from build123d import *

# Parameters (mm, degrees)
ESQUISSE1_W        = 30
ESQUISSE1_H        = 140
ESQUISSE1_H_2      = 30
ESQUISSE1_W_2      = 350
BOSS_EXTRU_1_DEPTH = 580


with BuildPart() as part:
    # Esquisse1 → Boss.-Extru.1 (new body)
    with BuildSketch(Plane.XY):
        with Locations((-15, 100)):
            Rectangle(ESQUISSE1_W, ESQUISSE1_H)
        with Locations((-15, 15)):
            Rectangle(ESQUISSE1_W, ESQUISSE1_H_2)
        with Locations((175, 15)):
            Rectangle(ESQUISSE1_W_2, ESQUISSE1_H_2)
        with Locations((365, 15)):
            Rectangle(ESQUISSE1_W, ESQUISSE1_H_2)
        with Locations((365, 100)):
            Rectangle(ESQUISSE1_W, ESQUISSE1_H)
        Polygon((-30, 170), (-30, 152.681524316), (-15, 161.340762158), align=None)
        Polygon((-15, 161.340762158), (0, 170), (-30, 170), align=None)
        Polygon((-15, 161.340762158), (0, 152.681524316), (0, 170), align=None)
        Polygon((380, 170), (350, 170), (380, 152.681524316), align=None)
    extrude(amount=BOSS_EXTRU_1_DEPTH)


solid = part.part
Source: CAD feature listing. Evaluate the final solid. Frame: model axes, mm. A direction names the side the tool comes from. Coordinates: 2 decimals unless noted, no trailing zeros. Loops run counter-clockwise (first coordinate to the right, second up) from the corner with the lowest first, then second, coordinate; pieces in that order, holes last. Notation, with made-up numbers: (73.25, 7.25) - (99.25, 7.25) arc R7 ccw to (99.25, 13.25) - close; hole circle Ø1 at (62.25, 89.25). An arc over 180 degrees is marked (long way). One line per item, written item: value. Start each with the question number.
1. Contact query for flat-ended pins moving along their axis: P1, Ø3, axis at x = 118, z = 443.5, coming from the -Y side; P2, Ø6, axis at x = 302, z = 151, coming from the +Y side; P3, Ø10, axis at x = 25.5, y = 36, coming from the +Z side. Output: stop coordinate, or through.
2. Set-up query: faces 1 (the flat face through (365, 170, 286)), 2 (the flat face through (177, 30, 286)). Return all of +Z, -Z, +X, -X, +Y, -Y with unobstructed straight access to the full face (end or side cutting, diameter ignored); none if empty.
3. Section C-C (x = 108.5). Return the cut outline in (y, z), and give its area (3 significant figures).
4. Ray query, L1, parallel to X at y = 68, z = 544.5; L2, parallel to Y at x = 196.5, z = 182. Return the intervals inside material, ascending.
5. Section A-A (y = 139). Return the cut outline in (x, z), and give its area (3 significant figures).
6. Section B-B (z = 335). Return the cut outline in (x, y), and give its area (3 significant figures).
Verdict:
1. P1: stops at y = 0
1. P2: stops at y = 30
1. P3: passes through
2. face 1: +Z, -Z, +X, -X, +Y
2. face 2: +Z, -Z, +Y
3. outline: (0, 0) - (30, 0) - (30, 580) - (0, 580) - close
3. area: 17,400 mm2
4. L1: x = -30 to 0, 350 to 380
4. L2: y = 0 to 30
5. outline: (-30, 0) - (0, 0) - (0, 580) - (-30, 580) - close; (350, 0) - (380, 0) - (380, 580) - (350, 580) - close
5. area: 34,800 mm2
6. outline: (-30, 0) - (380, 0) - (380, 170) - (350, 170) - (350, 30) - (0, 30) - (0, 170) - (-30, 170) - close
6. area: 20,700 mm2
